Build history of the part. All positions in model axes, mm. Face numbers are marked on the shaded views. A direction names the side the tool comes from. Round coordinates to 2 decimals unless told otherwise and drop trailing zeros. Order: outer loops, then holes, each group sorted by start corner. A loop starts at its lowest first (then second) coordinate and runs counter-clockwise, first axis right, second up. Notation, with made-up numbers: (60.5, 30) -> (115.5, 30) arc R32 cw to (115.5, 62) -> close; hole circle Ø1 at (-19.5, 39.25). An arc over 180 degrees is marked (long way). Use a Markdown table: item, result. Add a question column.
Item 1: Pin check, flat tips, straight feed: pin 1 (1.5 mm diameter, centred on x = -1, z = 5, fed in from +Y); pin 2 (1.5 mm diameter, centred on x = -4, z = 4, fed in from +Y); pin 3 (1.5 mm diameter, centred on x = -0.5, z = 2.5, fed in from -Y). Stop position of each tip, or through.
Item 2: Slice it at C-C, the plane z = 1.25. Give the cut face in (x, y).
Item 3: Probe L1, parallel to Z at x = 6.75, y = 0.25; L2, parallel to Y at x = -9, z = 2; L3, parallel to Y at x = 0.75, z = 3. List the from-to ranges inside material, lowest first.
Item 4: Slice it at A-A, the plane x = 0. Give the cut face in (y, z).
Item 5: 3-axis set-ups, long thin cutter, end or side, ignore diameter. For the marked faces 1 and 2: which of +Z, -Z, +X, -X, +Y, -Y reach the whole face in a straight line?
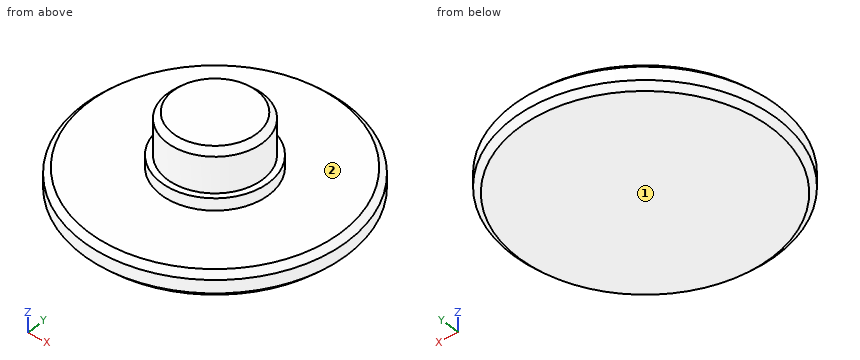
from build123d import *

# Parameters (mm, degrees)
F0_R     = 11.05
F1_DEPTH = 2.1
F2_R     = 4.5
F3_DEPTH = 1.01
F4_R     = 3.99
F5_DEPTH = 3.5
F6_SIZE  = 0.5


with BuildPart() as f1:
    # F0 (on Top) → F1 (new body)
    with BuildSketch(Plane.XY):
        Circle(F0_R)
    extrude(amount=F1_DEPTH)

    # F2 (on face) → F3 (join)
    with BuildSketch(Plane.XY.offset(2.1)):
        Circle(F2_R)
    extrude(amount=F3_DEPTH)

    # F4 (on face) → F5 (join)
    with BuildSketch(Plane.XY.offset(3.11)):
        Circle(F4_R)
    extrude(amount=F5_DEPTH)

    # F6
    f6_edges = [f1.edges().sort_by_distance(p)[0] for p in [
        (-11.05, 0, 2.1),
        (-3.99, 0, 6.61),
        (-11.05, 0, 0),
    ]]
    chamfer(f6_edges, length=F6_SIZE)


solid = f1.part
Check sheet entries:
| question | item | result |
|---|---|---|
| 1 | pin 1 | y = 3.98 |
| 1 | pin 2 | y = 2.31 |
| 1 | pin 3 | y = -10.89 |
| 2 | outline | circle Ø22.1 at (0, 0) |
| 3 | L1 | 0 to 2.1 |
| 3 | L2 | -5.69 to 5.69 |
| 3 | L3 | -4.44 to 4.44 |
| 4 | outline | (-11.05, 0.5) -> (-10.55, 0) -> (10.55, 0) -> (11.05, 0.5) -> (11.05, 1.6) -> (10.55, 2.1) -> (4.5, 2.1) -> (4.5, 3.11) -> (3.99, 3.11) -> (3.99, 6.11) -> (3.49, 6.61) -> (-3.49, 6.61) -> (-3.99, 6.11) -> (-3.99, 3.11) -> (-4.5, 3.11) -> (-4.5, 2.1) -> (-10.55, 2.1) -> (-11.05, 1.6) -> close |
| 5 | face 1 | -Z, +X, -X, +Y, -Y |
| 5 | face 2 | +Z |
